Geometry: final body of the model. Coordinates: model frame, mm. A direction names the side the tool comes from. Give positions to 0.01 mm unless a question says otherwise; leave off trailing zeros. Loops run counter-clockwise (first coordinate to the right, second up) from the corner with the lowest first, then second, coordinate; pieces in that order, holes last. Notation, with made-up numbers: (53, -22) - (72, -22) arc R16 ccw to (72, 0) - close; hole circle Ø9 at (65, 20.25). An arc over 180 degrees is marked (long way). Use one line per item in the form item = value.
```python
from build123d import *

# Parameters (mm, degrees)
SKETCH1_R                = 5
BOSS_EXTRUDE1_DEPTH      = 35
BOSS_EXTRUDE5_DEPTH      = 60
BOSS_EXTRUDE5_DEPTH_BACK = 5
SKETCH2_R                = 4.7625
CHAMFER1_SIZE            = 1


with BuildPart() as part:
    # Sketch1 → Boss-Extrude1 (new, symmetric)
    with BuildSketch(Plane(origin=(0, 0, 0), x_dir=(0, 0, -1), z_dir=(1, 0, 0))):
        with Locations((0, -5)):
            Circle(SKETCH1_R)
    extrude(amount=BOSS_EXTRUDE1_DEPTH, both=True)

    # Sketch2 → Boss-Extrude5 (add, two sides: drawn at the far end of the back side and taken through both)
    with BuildSketch(Plane(origin=(0, 0, 0), x_dir=(1, 0, 0), z_dir=(0, 1, 0)).offset(-BOSS_EXTRUDE5_DEPTH_BACK)):
        with Locations(Location((0, 0, 0), (0, 0, 270))):
            Circle(SKETCH2_R)
    extrude(amount=BOSS_EXTRUDE5_DEPTH + BOSS_EXTRUDE5_DEPTH_BACK)

    # Chamfer1
    chamfer1_edges = [part.edges().sort_by_distance(p)[0] for p in [
        (-35, -5, 5),
        (35, -5, 5),
        (0, 60, -4.7625),
    ]]
    chamfer(chamfer1_edges, length=CHAMFER1_SIZE)


solid = part.part
```
(1) Access query for faces 1 (the face through (0.476, -9.436, -2.307)), 2 (the face through (1.431, 27.324, 4.543)), 3 (the face through (0, 60, 0)). Directions: +Z, -Z, +X, -X, +Y, -Y. A direction counts if a zero-diameter tool reaches every point of the face in a straight line with its end or side. Return the directions, or none.
Solution:
face_1 = none
face_2 = +Y
face_3 = +Z, -Z, +X, -X, +Y
(2) Cut plane C-C (y = 18.5). Return the cut outline in (x, z) (1 decimal).
Solution:
outline = circle Ø9.5 at (0, 0)
(3) Cut plane A-A (x = 0). Return the cut outline in (y, z), plus the area to 3 significant figures.
Solution:
outline = (-3.48, -4.76) - (59, -4.76) - (60, -3.76) - (60, 3.76) - (59, 4.76) - (-3.48, 4.76) arc R5 ccw (long way) to start
area = 658 mm2
(4) Cut plane B-B (z = 0). Return the cut outline in (x, y), plus the area to 3 significant figures.
Solution:
outline = (-35, -9) - (-34, -10) - (34, -10) - (35, -9) - (35, -1) - (34, 0) - (4.76, 0) - (4.76, 59) - (3.76, 60) - (-3.76, 60) - (-4.76, 59) - (-4.76, 0) - (-34, 0) - (-35, -1) - close
area = 1,270 mm2
(5) Material intervals for L1, parallel to Z at x = 0, y = 50.5; L2, parallel to X at y = 54, z = -1.25; L3, parallel to Y at x = -22.5, z = 2.75, sorted ascending. Write a range as from..to.
Solution:
L1 = -4.76..4.76
L2 = -4.6..4.6
L3 = -9.18..-0.82
(6) Cut plane D-D (x = 27.5). Return the cut outline in (y, z), plus the area to 3 significant figures.
Solution:
outline = circle Ø10 at (-5, 0)
area = 78.5 mm2
(7) Pin query (flat end, axial travel): P1, Ø6, axis at x = -17.5, z = -3, coming from the +Y side; P2, Ø2, axis at y = 50.5, z = 2, coming from the +X side; P3, Ø1.5, axis at x = -26, z = -1.5, coming from the +Y side. Return the tip coordinate at first contact, or that it passes through.
Solution:
P1 = 0
P2 = 4.66
P3 = -0.06
